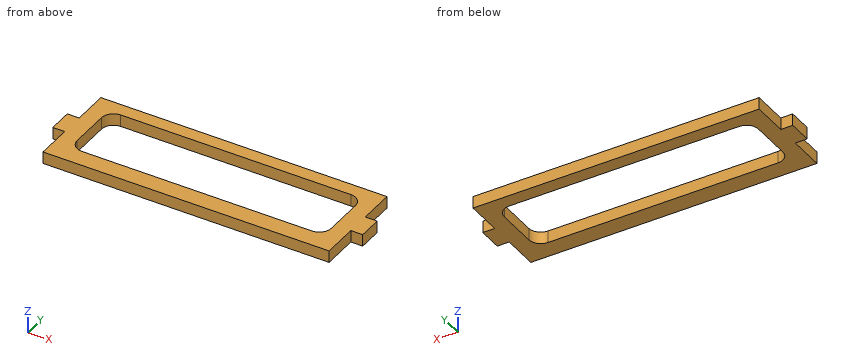
from build123d import *

# Parameters (mm, degrees)
F1_DEPTH = 5
F3_DEPTH = 25


with BuildPart() as f1:
    # F0 (on Top) → F1 (new body)
    with BuildSketch(Plane.XY):
        Polygon((47.113799, 25), (-72.886201, 25), (-72.886201, 10), (-77.886201, 10), (-77.886201, 0), (-72.886201, 0), (-72.886201, -15), (47.113799, -15), (47.113799, 0), (52.113799, 0), (52.113799, 10), (47.113799, 10), align=None)
        with BuildLine():
            ThreePointArc((-62.401845, 10.947084), (-60.937379, 14.482618), (-57.401845, 15.947084))
            Line((-57.401845, 15.947084), (-27.401845, 15.947084))
            ThreePointArc((-27.401845, 15.947084), (-25.855638, 15.702002), (-24.46101, 14.990782))
            ThreePointArc((-24.46101, 14.990782), (-22.946277, 13.215985), (-22.401845, 10.947084))
            Line((-22.401845, 10.947084), (-22.401845, 0.947084))
            ThreePointArc((-22.401845, 0.947084), (-23.866311, -2.58845), (-27.401845, -4.052916))
            Line((-27.401845, -4.052916), (-57.401845, -4.052916))
            ThreePointArc((-57.401845, -4.052916), (-60.937379, -2.58845), (-62.401845, 0.947084))
            Line((-62.401845, 0.947084), (-62.401845, 10.947084))
        make_face(mode=Mode.SUBTRACT)
        with BuildLine():
            ThreePointArc((2.598155, -4.052916), (-0.937379, -2.58845), (-2.401845, 0.947084))
            Line((-2.401845, 0.947084), (-2.401845, 10.947084))
            ThreePointArc((-2.401845, 10.947084), (-0.937379, 14.482618), (2.598155, 15.947084))
            Line((2.598155, 15.947084), (32.598155, 15.947084))
            ThreePointArc((32.598155, 15.947084), (36.133689, 14.482618), (37.598155, 10.947084))
            Line((37.598155, 10.947084), (37.598155, 0.947084))
            ThreePointArc((37.598155, 0.947084), (36.133689, -2.58845), (32.598155, -4.052916))
            Line((32.598155, -4.052916), (2.598155, -4.052916))
        make_face(mode=Mode.SUBTRACT)
    extrude(amount=F1_DEPTH)

    # F2 (on face) → F3 (cut)
    with BuildSketch(Plane.XY.offset(5)):
        with BuildLine():
            ThreePointArc((40.378798, 14.351363), (38.914332, 17.886897), (35.378798, 19.351363))
            Line((35.378798, 19.351363), (-61.151201, 19.351363))
            ThreePointArc((-61.151201, 19.351363), (-64.686735, 17.886897), (-66.151201, 14.351363))
            Line((-66.151201, 14.351363), (-66.151201, -2.457194))
            ThreePointArc((-66.151201, -2.457194), (-64.686735, -5.992728), (-61.151201, -7.457194))
            Line((-61.151201, -7.457194), (35.378798, -7.457194))
            ThreePointArc((35.378798, -7.457194), (38.914332, -5.992728), (40.378798, -2.457194))
            Line((40.378798, -2.457194), (40.378798, 14.351363))
        make_face()
        with BuildLine():
            ThreePointArc((-57.401845, -4.052916), (-60.937379, -2.58845), (-62.401845, 0.947084))
            Line((-62.401845, 0.947084), (-62.401845, 10.947084))
            ThreePointArc((-62.401845, 10.947084), (-60.937379, 14.482618), (-57.401845, 15.947084))
            Line((-57.401845, 15.947084), (-27.401845, 15.947084))
            ThreePointArc((-27.401845, 15.947084), (-23.866311, 14.482618), (-22.401845, 10.947084))
            Line((-22.401845, 10.947084), (-22.401845, 0.947084))
            ThreePointArc((-22.401845, 0.947084), (-23.866311, -2.58845), (-27.401845, -4.052916))
            Line((-27.401845, -4.052916), (-57.401845, -4.052916))
        make_face(mode=Mode.SUBTRACT)
        with BuildLine():
            ThreePointArc((37.598155, 0.947084), (36.133689, -2.58845), (32.598155, -4.052916))
            Line((32.598155, -4.052916), (2.598155, -4.052916))
            ThreePointArc((2.598155, -4.052916), (-0.937379, -2.58845), (-2.401845, 0.947084))
            Line((-2.401845, 0.947084), (-2.401845, 10.947084))
            ThreePointArc((-2.401845, 10.947084), (-0.937379, 14.482618), (2.598155, 15.947084))
            Line((2.598155, 15.947084), (32.598155, 15.947084))
            ThreePointArc((32.598155, 15.947084), (36.133689, 14.482618), (37.598155, 10.947084))
            Line((37.598155, 10.947084), (37.598155, 0.947084))
        make_face(mode=Mode.SUBTRACT)
    extrude(amount=-F3_DEPTH, mode=Mode.SUBTRACT)


solid = f1.part
The model under review builds one solid part; all positions refer to its coordinate system, in mm. Coordinates: 2 decimals unless noted, no trailing zeros. Loops run counter-clockwise (first coordinate to the right, second up) from the corner with the lowest first, then second, coordinate; pieces in that order, holes last. Notation, with made-up numbers: M 50,80 L 64,80 A17 ccw 64,89 Z; hole C -13,-7 d11. An arc over 180 degrees is marked long. Put each result on its own line as item: value. Start each with the question number.
Q1. Add section B-B (x = 6). Write out the cut boundary in (y, z).
Q2. Add section C-C (z = 1.5). Write out the cut boundary in (x, y), and give its area (3 significant figures).
Q3. Add section A-A (y = 8). Write out the cut boundary in (x, z).
Q4. Wall thickness on line 1 (Y direction, x = 24, z = 4.25); line 2 (Y direction, x = -61.5, z = 3.5); line 3 (X direction, y = 13, z = 2.8): over which ranges is each line inside the solid? List them lowest first.
Q5. Add section D-D (y = -10). Write out the cut boundary in (x, z), and give its area (3 significant figures).
Q6. Clearance check with a flat-ended pin moving along its axis: pin 1 (2.5 mm diameter, centred on x = 50, z = 3, fed in from +Y). State where the tip first meets the part, or that it passes through.
Answers:
1. outline: M -15,0 L -7.46,0 L -7.46,5 L -15,5 Z; M 19.35,0 L 25,0 L 25,5 L 19.35,5 Z
2. outline: M -77.89,0 L -72.89,0 L -72.89,-15 L 47.11,-15 L 47.11,0 L 52.11,0 L 52.11,10 L 47.11,10 L 47.11,25 L -72.89,25 L -72.89,10 L -77.89,10 Z; hole M -66.15,-2.46 A5 ccw -61.15,-7.46 L 35.38,-7.46 A5 ccw 40.38,-2.46 L 40.38,14.35 A5 ccw 35.38,19.35 L -61.15,19.35 A5 ccw -66.15,14.35 Z
2. area: 2,070 mm^2
3. outline: M -77.89,0 L -66.15,0 L -66.15,5 L -77.89,5 Z; M 40.38,0 L 52.11,0 L 52.11,5 L 40.38,5 Z
4. line 1: y = -15 to -7.46, 19.35 to 25
4. line 2: y = -15 to -7.45, 19.34 to 25
4. line 3: x = -72.89 to -66.15, 40.38 to 47.11
5. outline: M -72.89,0 L 47.11,0 L 47.11,5 L -72.89,5 Z
5. area: 600 mm^2
6. pin 1: stops at y = 10
